Part model, mm, in its own coordinate system. Round coordinates to 2 decimals unless told otherwise and drop trailing zeros. Write each loop counter-clockwise with the first axis right and the second up, starting at its lowest first coordinate (ties: lowest second). Pieces come first, ordered by that corner, then holes. Notation, with made-up numbers: (-31.75, -16.75) -> (-23.75, -16.75) arc R32 ccw to (-23.75, 18.25) -> close; hole circle Ø10 at (79.25, 4.25). An arc over 180 degrees is marked (long way). Return JSON: item names as keys, results as strings. Group by question number.
(1) Drill centre lines: L1, parallel to Z at x = 241.5, y = -3.25; L2, parallel to X at y = 0, z = -661.5; L3, parallel to X at y = 4, z = -70.5. Where is each one in solid material? Low to high. Write a range as from..to.
(2) Drop flat-ended pins along their axis: pin 1 Ø3 at (x, y) = (168.5, -2) entering from +Z; pin 2 Ø8.5 at (y, z) = (-3.5, -19.5) entering from +X; pin 3 Ø10 at (x, y) = (132, -3.5) entering from -Z. Give the stop position or say it passes through.
(3) Saw through at A-A (y = 3.75). List the corners of the cut face in (x, z), plus the area to 3 significant figures.
from build123d import *

# Parameters (mm, degrees)
SKETCH1_W           = 1219.2
SKETCH1_H           = 1771.65
BOSS_EXTRUDE1_DEPTH = 9.525
SKETCH3_W           = 184.1373
SKETCH3_H           = 76.2
SKETCH3_W_2         = 88.9
SKETCH3_W_3         = 179.3875
SKETCH3_W_4         = 15.2273
CUT_EXTRUDE2_DEPTH  = 20.05
CHAMFER1_SIZE       = 2.54


with BuildPart() as part:
    # Sketch1 → Boss-Extrude1 (new body, symmetric)
    with BuildSketch(Plane(origin=(0, 0, 0), x_dir=(1, 0, 0), z_dir=(0, 1, 0))):
        with Locations((609.6, 885.825)):
            Rectangle(SKETCH1_W, SKETCH1_H)
    extrude(amount=BOSS_EXTRUDE1_DEPTH, both=True)

    # Sketch3 → Cut-Extrude2 (cut, through all)
    with BuildSketch(Plane(origin=(0, 9.525, 0), x_dir=(1, 0, 0), z_dir=(0, 1, 0))):
        with Locations((173.78045, 1733.55)):
            Rectangle(SKETCH3_W, SKETCH3_H)
        with Locations((1174.75, 1733.55)):
            Rectangle(SKETCH3_W_2, SKETCH3_H)
        Polygon((84.1756, 684.212499999), (173.167165563, 684.212499999), (173.167165563, 646.125199999), (263.5631, 646.125199999), (263.5631, 608.012499999), (84.1756, 608.012499999), align=None)
        with Locations((173.86935, 38.1)):
            Rectangle(SKETCH3_W_3, SKETCH3_H)
        with Locations((1174.75, 38.1)):
            Rectangle(SKETCH3_W_2, SKETCH3_H)
        with Locations((7.61365, 1733.55)):
            Rectangle(SKETCH3_W_4, SKETCH3_H)
    extrude(amount=-CUT_EXTRUDE2_DEPTH, mode=Mode.SUBTRACT)

    # Chamfer1
    chamfer1_edges = [part.edges().sort_by_distance(p)[0] for p in [
        (0, 9.525, -847.725),
        (696.93155, 9.525, 0),
        (1219.2, 9.525, -885.825),
        (698.07455, 9.525, -1771.65),
        (48.46955, 9.525, -1771.65),
        (7.61365, 9.525, -1695.45),
        (15.2273, 9.525, -1733.55),
        (1174.75, 9.525, -76.2),
        (1130.3, 9.525, -38.1),
        (263.5631, 9.525, -38.1),
        (173.86935, 9.525, -76.2),
        (84.1756, 9.525, -38.1),
        (84.1756, 9.525, -646.112499999),
        (173.86935, 9.525, -608.012499999),
        (263.5631, 9.525, -627.068849999),
        (218.365132782, 9.525, -646.125199999),
        (173.167165563, 9.525, -665.168849999),
        (128.671382782, 9.525, -684.212499999),
        (1130.3, 9.525, -1733.55),
        (1174.75, 9.525, -1695.45),
        (81.7118, 9.525, -1733.55),
        (173.78045, 9.525, -1695.45),
        (265.8491, 9.525, -1733.55),
        (42.0878, 9.525, 0),
    ]]
    chamfer(chamfer1_edges, length=CHAMFER1_SIZE)


solid = part.part
Computed values:
{
 "1": {"L1": "-1695.45..-646.13, -608.01..-76.2", "L2": "0..84.18, 173.17..1219.2", "L3": "0..84.18, 263.56..1130.3"},
 "2": {"pin 1": "z = -76.2", "pin 2": "x = 1130.3", "pin 3": "z = -1695.45"},
 "3": {"outline": "(0, -1695.45) -> (15.23, -1695.45) -> (15.23, -1771.65) -> (81.71, -1771.65) -> (81.71, -1695.45) -> (265.85, -1695.45) -> (265.85, -1771.65) -> (1130.3, -1771.65) -> (1130.3, -1695.45) -> (1219.2, -1695.45) -> (1219.2, -76.2) -> (1130.3, -76.2) -> (1130.3, 0) -> (263.56, 0) -> (263.56, -76.2) -> (84.18, -76.2) -> (84.18, 0) -> (0, 0) -> close; hole (84.18, -684.21) -> (173.17, -684.21) -> (173.17, -646.13) -> (263.56, -646.13) -> (263.56, -608.01) -> (84.18, -608.01) -> close", "area": "2,110,000 mm2"}
}
